Autodesk Inventor part; units mm, degrees
ref_plane "YZ Plane" through (0, 0, 0) normal (1, 0, 0) x (0, 1, 0)
ref_plane "XZ Plane" through (0, 0, 0) normal (0, 1, 0) x (-1, 0, 0)
ref_plane "XY Plane" through (0, 0, 0) normal (0, 0, 1) x (1, 0, 0)
sketch "Sketch1" plane through (0, 0, 0) normal (0, 0, 1) x (1, 0, 0)
  line L0 (0, 0) -> (-145.9112, 0)
  line L1 (-145.9112, 0) -> (-145.9112, -1500)
  line L2 (-145.9112, -1500) -> (0, -1500)
  line L3 (0, -1500) -> (0, 0)
  line L4 (-145.9112, -1400) -> (-81, -1400)
  line L5 (-81, -1400) -> (-81, -1394)
  line L6 (-81, -1394) -> (-145.9112, -1394)
  line L7 (-145.9112, -1394) -> (-145.9112, -1400)
  line L8 (-145.9112, -900) -> (-81, -900)
  line L9 (-81, -900) -> (-81, -894)
  line L10 (-81, -894) -> (-145.9112, -894)
  line L11 (-145.9112, -894) -> (-145.9112, -900)
  line L12 (-145.9112, -400) -> (-81, -400)
  line L13 (-81, -400) -> (-81, -394)
  line L14 (-81, -394) -> (-145.9112, -394)
  line L15 (-145.9112, -394) -> (-145.9112, -400)
  point P0 (-145.9112, -394)
  point P1 (-145.9112, -400)
  point P2 (-145.9112, -894)
  point P3 (-145.9112, -900)
  point P4 (-145.9112, -1394)
  dimension "d0" = 1500
  dimension "d1" = 145.9112
  dimension "d2" = 6
  dimension "d4" = 100
  dimension "d7" = 500
  dimension "d23" = 81
extrude "Plate1" add sketch "Sketch1" along normal blind 4 contours L3 L2 L1 L4 L5 L6 L8 L9 L10 L12 L13 L14 L0
sketch "Sketch2" plane through (4, 0, 0) normal (-1, 0, 0) x (0, -1, 0)
  line L0 (1500, 0) -> (0, 0)
  line L1 (0, 0) -> (0, 35)
  line L2 (0, 35) -> (1500, 35)
  line L3 (1500, 35) -> (1500, 0)
edge flange "Flange1" height 35 angle 90 thickness 4 bend radius 4 thickness toward (-1, 0, 0) relief tear relief width 4 relief depth 2 edges at (0, -750, 4) wall of the first edge with corners at (4, -1500, 0) (4, 0, 0) (4, 0, 35) (4, -1500, 35)
bend "Bend1"
corner "Corner1"
equation "\"d1\" = Stringer2_3_deep"
equation "\"d12\" = Thickness"
equation "\"d13\" = BendReliefWidth"
equation "\"d14\" = BendReliefDepth"
equation "\"d15\" = MinimumRemnant"
equation "\"d16\" = TransitionRadius"
equation "\"d19\" = BendRadius"
equation "\"d20\" = CornerReliefSize"
equation "\"d21\" = GapSize"
equation "\"d22\" = JacobiRadiusSize"
equation "\"BendRadius\" = Thickness"
equation "\"BendReliefWidth\" = Thickness"
equation "\"BendReliefDepth\" = 0.5 * Thickness"
equation "\"CornerReliefSize\" = 4 * Thickness"
equation "\"MinimumRemnant\" = 2 * Thickness"
equation "\"TransitionRadius\" = BendRadius"
equation "\"JacobiRadiusSize\" = BendRadius"
equation "\"GapSize\" = Thickness"
properties part number "stringer 1.3_CPY2"
Check sheet for the modelled part. Datum: model origin and axes. Units: mm. A direction names the side the tool comes from. Give positions to 0.01 mm unless a question says otherwise; leave off trailing zeros. Write each loop counter-clockwise with the first axis right and the second up, starting at its lowest first coordinate (ties: lowest second). Pieces come first, ordered by that corner, then holes.
Item 1: Scan lines: L1, parallel to Y at x = -138.5, z = 3.5; L2, parallel to Z at x = -65, y = -353.5. Record each from-to range of solid material in increasing order.
Item 2: Cross-section at A-A (x = -125). Enter the section's corners in (y, z).
Item 3: Cross-section at B-B (y = -1324). Enter the section's corners in (x, z), and give its area (3 significant figures).
Item 4: Gauge pin test, flat ends, axial feed: pin 1 (4 mm diameter, centred on x = -13.5, y = -1197, fed in from +Z); pin 2 (2 mm diameter, centred on y = -397, z = 2.5, fed in from -X); pin 3 (3 mm diameter, centred on y = -844.5, z = 8, fed in from -X). Record the tip position at first contact, or that the pin passes through.
Item 5: Cross-section at C-C (z = 20). Enter the section's corners in (x, y).
Item 6: Access from +Z, -Z, +X, -X, +Y, -Y to the whole of each face (thin tool, end or side, straight path). Record for faces 1 (the face through (0, -740, 21)), 2 (the face through (4, -740, 22)).
Item 7: Cross-section at D-D (x = -46). Enter the section's corners in (y, z), and give its area (3 significant figures).
Report:
1. L1: y = -1500 to -1400, -1394 to -900, -894 to -400, -394 to 0
1. L2: z = 0 to 4
2. outline: (-1500, 0) - (-1400, 0) - (-1400, 4) - (-1500, 4) - close; (-1394, 0) - (-900, 0) - (-900, 4) - (-1394, 4) - close; (-894, 0) - (-400, 0) - (-400, 4) - (-894, 4) - close; (-394, 0) - (0, 0) - (0, 4) - (-394, 4) - close
3. outline: (-145.91, 0) - (-4, 0) arc R8 ccw to (4, 8) - (4, 35) - (0, 35) - (0, 8) arc R4 cw to (-4, 4) - (-145.91, 4) - close
3. area: 713 mm2
4. pin 1: stops at z = 4
4. pin 2: stops at x = -81
4. pin 3: stops at x = -0.29
5. outline: (0, -1500) - (4, -1500) - (4, 0) - (0, 0) - close
6. face 1: +Z, -X, +Y, -Y
6. face 2: +Z, -Z, +X, +Y, -Y
7. outline: (-1500, 0) - (0, 0) - (0, 4) - (-1500, 4) - close
7. area: 6,000 mm2
